The model under review builds one solid part; all positions refer to its coordinate system, in mm. Coordinates: 2 decimals unless noted, no trailing zeros. Write each loop counter-clockwise with the first axis right and the second up, starting at its lowest first coordinate (ties: lowest second). Pieces come first, ordered by that corner, then holes.
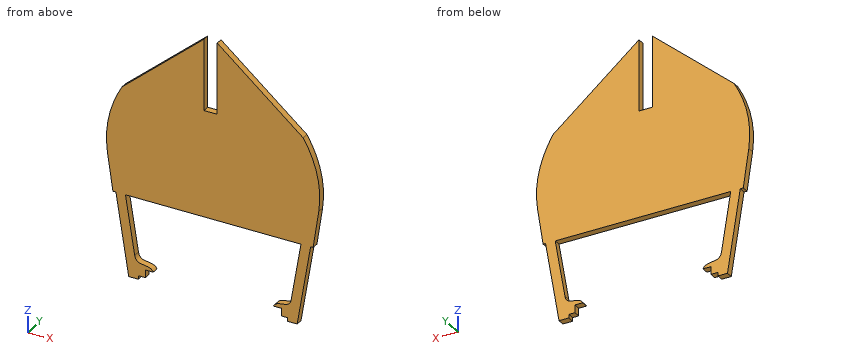
```python
from build123d import *

# Parameters (mm, degrees)
EXTRUDE_2_DEPTH = 4


with BuildPart() as part:
    # 草图1 → 凸台-拉伸2 (new body)
    with BuildSketch(Plane(origin=(0, 0, 0), x_dir=(1, 0, 0), z_dir=(0, 1, 0))):
        with BuildLine():
            Line((-7.493646731, 0), (-10.814865867, -22.617855932))
            add(Edge.make_bspline(
                [(-10.814865867, -22.617855932), (-13.583142705, -44.426344102), (-1.98899974, -64.01075601)],
                knots=[0, 0, 0, 1, 1, 1], degree=2))
            Line((-1.98899974, -64.01075601), (46.968083593, -106.186589343))
            Line((46.968083593, -106.186589343), (46.968083593, -63.586589343))
            Line((46.968083593, -63.586589343), (54.968083593, -63.586589343))
            Line((54.968083593, -63.586589343), (54.968083593, -106.186589343))
            Line((54.968083593, -106.186589343), (106.410598372, -64.01075601))
            add(Edge.make_bspline(
                [(115.792042318, -22.617855932), (118.672533556, -44.533714829), (106.410598372, -64.01075601)],
                knots=[0, 0, 0, 1, 1, 1], degree=2))
            Line((115.792042318, -22.617855932), (112.396356875, -0.121439872))
            Line((112.396356875, -0.121439872), (110.919371618, -0.121439872))
            Line((110.919371618, -0.121439872), (102.847231691, 48.365226521))
            Line((102.847231691, 48.365226521), (97.014954375, 48.365226521))
            Line((97.014954375, 48.365226521), (97.014954375, 46.231466528))
            Line((97.014954375, 46.231466528), (93.316437053, 46.231466528))
            Line((93.316437053, 46.231466528), (93.316437053, 41.625642308))
            Line((93.316437053, 41.625642308), (88.622165067, 41.625642308))
            add(Edge.make_bspline(
                [(88.622165067, 41.625642308), (91.029256543, 36.904254059), (98.571856956, 41.17808537), (99.290965035, 34.709162562)],
                knots=[0, 0, 0, 0, 1, 1, 1, 1], degree=3))
            Line((99.290965035, 34.709162562), (105.12324235, 0))
            Line((105.12324235, 0), (0, 0))
            Line((0, 0), (5.547775983, 34.709162562))
            add(Edge.make_bspline(
                [(16.649061602, 41.625642308), (14.296406024, 36.889271563), (6.70760812, 41.39847379), (5.547775983, 34.709162562)],
                knots=[0, 0, 0, 0, 1, 1, 1, 1], degree=3))
            Line((16.649061602, 41.625642308), (11.922711294, 41.625642308))
            Line((11.922711294, 41.625642308), (11.922711294, 46.231466528))
            Line((11.922711294, 46.231466528), (7.707317775, 46.231466528))
            Line((7.707317775, 46.231466528), (7.707317775, 48.365226521))
            Line((7.707317775, 48.365226521), (1.959053886, 48.365226521))
            Line((1.959053886, 48.365226521), (-5.705297966, 0))
            Line((-5.705297966, 0), (-7.493646731, 0))
        make_face()
    extrude(amount=EXTRUDE_2_DEPTH)


solid = part.part
```
Item 1: Take a section at B-B, the plane x = 51.5. Write out the cut boundary in (y, z), plus the area to 3 significant figures.
Solved:
outline: (0, 0) - (4, 0) - (4, 63.59) - (0, 63.59) - close
area: 254 mm2
Item 2: For pin 1 (2 mm diameter, centred on x = 21, y = 1.5, fed in from -Z); pin 2 (1.7 mm diameter, centred on y = 1, z = -47.5, fed in from -X); pin 3 (1.2 mm diameter, centred on y = 2, z = 94.5, fed in from -X), all flat-tipped, find the tip position at first contact; note any pin that passes through.
Solved:
pin 1: stops at z = 0
pin 2: stops at x = 1.69
pin 3: stops at x = 32.71
Item 3: To check wall thickness, follow line 1 along X through (y, z) = (3.4, 70.5); line 2 along X through (y, z) = (2.65, -7); line 3 along Z through (x, y) = (11, 2.05). State the ranges of each line that lie inside material, in increasing order.
Solved:
line 1: x = 5.54 to 46.97, 54.97 to 98.5
line 2: x = -4.6 to 1.12, 103.95 to 109.73
line 3: z = -46.23 to -38.94, 0 to 75.2
Item 4: Take a section at C-C, the plane z = 10.5. Write out the cut boundary in (x, y).
Solved:
outline: (-9.04, 0) - (113.96, 0) - (113.96, 4) - (-9.04, 4) - close
Item 5: Take a section at A-A, the plane z = -7.5. Write out the cut boundary in (x, y), plus the area to 3 significant figures.
Solved:
outline: (-4.52, 0) - (1.2, 0) - (1.2, 4) - (-4.52, 4) - close; (103.86, 0) - (109.65, 0) - (109.65, 4) - (103.86, 4) - close
area: 46.0 mm2
